```python
from build123d import *

# Parameters (mm, degrees)
SKETCH1_R           = 11
BOSS_EXTRUDE1_DEPTH = 47.2
SKETCH2_W           = 1
SKETCH2_H           = 5
SKETCH3_W           = 2.3
SKETCH3_H           = 3
SKETCH4_R           = 1.5
BOSS_EXTRUDE2_DEPTH = 9
SKETCH5_R           = 1
BOSS_EXTRUDE3_DEPTH = 2.65


with BuildPart() as part:
    # Sketch1 → Boss-Extrude1 (new body)
    with BuildSketch(Plane.XY):
        Circle(SKETCH1_R)
    extrude(amount=BOSS_EXTRUDE1_DEPTH)

    # Sketch2 → Revolve1 (revolve)
    with BuildSketch(Plane(origin=(0, 0, 0), x_dir=(0, 0, -1), z_dir=(1, 0, 0)), mode=Mode.PRIVATE) as revolve1_sk:
        with Locations((-47.7, 2.5)):
            Rectangle(SKETCH2_W, SKETCH2_H)
    revolve(revolve1_sk.sketch.rotate(Axis((0, 0, 47.2), (0, 0, -1)), 90), axis=Axis((0, 0, 47.2), (0, 0, -1)))

    # Sketch3 → Revolve2 (revolve)
    with BuildSketch(Plane(origin=(0, 0, 0), x_dir=(0, 0, -1), z_dir=(1, 0, 0)), mode=Mode.PRIVATE) as revolve2_sk:
        with Locations((1.15, 1.5)):
            Rectangle(SKETCH3_W, SKETCH3_H)
    revolve(revolve2_sk.sketch.rotate(Axis((0, 0, 47.2), (0, 0, -1)), 90), axis=Axis((0, 0, 47.2), (0, 0, -1)))

    # Sketch4 → Boss-Extrude2 (add)
    with BuildSketch(Plane.XY.offset(48.2)):
        Circle(SKETCH4_R)
    extrude(amount=BOSS_EXTRUDE2_DEPTH)

    # Sketch5 → Boss-Extrude3 (add)
    with BuildSketch(Plane(origin=(0, 0, -2.3), x_dir=(-1, 0, 0), z_dir=(0, 0, -1))):
        Circle(SKETCH5_R)
    extrude(amount=BOSS_EXTRUDE3_DEPTH)


solid = part.part
```
Can you work these out from the model? Positions are in its coordinate system, mm. A direction names the side the tool comes from. Coordinates: 2 decimals unless noted, no trailing zeros. Loops run counter-clockwise (first coordinate to the right, second up) from the corner with the lowest first, then second, coordinate; pieces in that order, holes last. Notation, with made-up numbers: (-28.5, -36.5) -> (-9.5, -36.5) arc R17 cw to (-9.5, -21.5) -> close; hole circle Ø3 at (85.5, -34). An arc over 180 degrees is marked (long way). Answer as a JSON object with one key per item and string values.
1) For faces 1 (the face through (-5, 0, 48)), 2 (the face through (0, -1, -4)), 3 (the face through (0, 0, 57.2)), which set-ups out of +Z, -Z, +X, -X, +Y, -Y let a thin tool reach every point of the face, with its end or its side?
Results:
{"face 1": "+Z", "face 2": "-Z", "face 3": "+Z, +X, -X, +Y, -Y"}
2) Imagine slicing it at C-C (z = 16). Please give me the cut outline in (x, y).
Results:
{"outline": "circle Ø22 at (0, 0)"}
3) Imagine slicing it at A-A (y = 0). Please give me the cut outline in (x, z).
Results:
{"outline": "(-11, 0) -> (-3, 0) -> (-3, -2.3) -> (-1, -2.3) -> (-1, -4.95) -> (1, -4.95) -> (1, -2.3) -> (3, -2.3) -> (3, 0) -> (11, 0) -> (11, 47.2) -> (5, 47.2) -> (5, 48.2) -> (1.5, 48.2) -> (1.5, 57.2) -> (-1.5, 57.2) -> (-1.5, 48.2) -> (-5, 48.2) -> (-5, 47.2) -> (-11, 47.2) -> close"}
4) Imagine slicing it at D-D (y = -4). Please give me the cut outline in (x, z).
Results:
{"outline": "(-10.25, 0) -> (10.25, 0) -> (10.25, 47.2) -> (3, 47.2) -> (3, 48.2) -> (-3, 48.2) -> (-3, 47.2) -> (-10.25, 47.2) -> close"}
5) If I drill on line 1 (Z direction, x = 7.5, y = 6.25); line 2 (Y direction, x = -0.5, z = 44); line 3 (Z direction, x = -1.75, y = -1), over which ranges is the centre line in solid material (lowest first)?
Results:
{"line 1": "z = 0 to 47.2", "line 2": "y = -10.99 to 10.99", "line 3": "z = -2.3 to 48.2"}
6) For P1, Ø5, axis at x = -7.5, z = 27.5, coming from the +Y side; P2, Ø1, axis at x = 3.5, y = 0.5, coming from the +Z side; P3, Ø4, axis at x = 8.5, y = 4, coming from the -Z side, each with a flat end and sliding along its axis, tell me the tip position at first contact or that it passes through.
Results:
{"P1": "stops at y = 9.8", "P2": "stops at z = 48.2", "P3": "stops at z = 0"}
